```python
from build123d import *

# Parameters (mm, degrees)
F1_DEPTH = 20


with BuildPart() as f1:
    # F0 (on Front) → F1 (new body)
    with BuildSketch(Plane.XZ):
        with BuildLine():
            ThreePointArc((-2.99453, 18.906719), (-4.468703, 18.613488), (-5.915325, 18.205498))
            ThreePointArc((-5.915325, 18.205498), (-11.251617, -15.486522), (19.142393, 0))
            ThreePointArc((19.142393, 0), (13.535716, 13.535716), (0, 19.142393))
            ThreePointArc((0, 19.142393), (-1.501895, 19.083384), (-2.99453, 18.906719))
        make_face()
        with BuildLine():
            Line((-6.445802, 19.838138), (-5.915325, 18.205498))
            ThreePointArc((-5.915325, 18.205498), (-4.468703, 18.613488), (-2.99453, 18.906719))
            Line((-2.99453, 18.906719), (-4.078854, 25.752868))
            Line((-4.078854, 25.752868), (-4.875689, 25.613901))
            ThreePointArc((-4.875689, 25.613901), (-5.214191, 25.41757), (-5.356509, 25.053049))
            Line((-5.356509, 25.053049), (-5.443327, 22.582582))
            Line((-5.443327, 22.582582), (-5.5143, 20.551845))
            ThreePointArc((-5.5143, 20.551845), (-5.633033, 20.215337), (-5.923472, 20.00802))
            Line((-5.923472, 20.00802), (-6.445802, 19.838138))
        make_face()
        with BuildLine():
            Line((-4.078854, 25.752868), (-2.99453, 18.906719))
            ThreePointArc((-2.99453, 18.906719), (-1.501895, 19.083384), (0, 19.142393))
            Line((0, 19.142393), (0, 20.859053))
            Line((0, 20.859053), (-0.549261, 20.859211))
            ThreePointArc((-0.549261, 20.859211), (-0.88955, 20.966631), (-1.106458, 21.249979))
            Line((-1.106458, 21.249979), (-1.80149, 23.159393))
            Line((-1.80149, 23.159393), (-2.647475, 25.482118))
            ThreePointArc((-2.647475, 25.482118), (-2.895471, 25.784819), (-3.278075, 25.866939))
            Line((-3.278075, 25.866939), (-4.078854, 25.752868))
        make_face()
    extrude(amount=F1_DEPTH)


solid = f1.part
```
Input: part model. Units: mm. Frame: model coordinates. Coordinates: 2 decimals unless noted, no trailing zeros. Order: outer loops, then holes, each group sorted by start corner. A loop starts at its lowest first (then second) coordinate and runs counter-clockwise, first axis right, second up. Notation, with made-up numbers: (-34.75, -17) - (-29.75, -17) arc R10 ccw to (-29.75, -12) - close; hole circle Ø8 at (-6.5, 45). An arc over 180 degrees is marked (long way). Return JSON: item names as keys, results as strings.
Q1. Cut plane C-C (z = 3.5). Return loops of the section in (x, y), then the cut area to 3 significant figures.
The answers:
{"outline": "(-18.82, -20) - (18.82, -20) - (18.82, 0) - (-18.82, 0) - close", "area": "753 mm2"}
Q2. Cut plane B-B (x = 1.5). Return loops of the section in (y, z).
The answers:
{"outline": "(-20, -19.08) - (0, -19.08) - (0, 19.08) - (-20, 19.08) - close"}
Q3. Draft query along Z for faces 1 (the flat face through (0, -10, 20)), 2 (the flat face through (-6.184, -9.86, 19.033)). Return one class per face: +Z half, -Z half, draft (parallel to the pull), parting line (faces both ways), or undercut.
The answers:
{"face 1": "draft", "face 2": "undercut"}
Q4. Cut plane A-A (y = -8). Return loops of the section in (x, z).
The answers:
{"outline": "(-6.45, 19.84) - (-5.92, 18.21) arc R19.14 ccw (long way) to (0, 19.14) - (0, 20.86) - (-0.55, 20.86) arc R0.59 cw to (-1.11, 21.25) - (-1.8, 23.16) - (-2.65, 25.48) arc R0.59 ccw to (-3.28, 25.87) - (-4.08, 25.75) - (-4.88, 25.61) arc R0.59 ccw to (-5.36, 25.05) - (-5.44, 22.58) - (-5.51, 20.55) arc R0.59 cw to (-5.92, 20.01) - close"}
Q5. First-contact query: pin 1 (12 mm diameter, centred on y = -6.5, z = 11, fed in from -X); pin 2 (6 mm diameter, centred on y = -11, z = 4, fed in from +X); pin 3 (4 mm diameter, centred on x = 13, y = -5, fed in from +Z). Flat tips, straight axial feed; report the tip coordinate or a pass-through.
The answers:
{"pin 1": "stops at x = -18.48", "pin 2": "stops at x = 19.12", "pin 3": "stops at z = 15.67"}
Q6. Ray query, probe 1 along Z at (x, y) = (0.5, -12.25); probe 2 along Z at (x, y) = (-0.5, -6.25). Return the intervals inside material, ascending.
The answers:
{"probe 1": "z = -19.14 to 19.14", "probe 2": "z = -19.14 to 20.86"}
